from build123d import *

# Parameters (mm, degrees)
SKETCH_1_W          = 210
SKETCH_1_H          = 70
EXTRUDE_1_DEPTH     = 8
SKETCH_2_W          = 190
SKETCH_2_H          = 60
CUT_EXTRUDE_1_DEPTH = 10
SKETCH_3_R          = 1.5
CUT_EXTRUDE_2_DEPTH = 10
SKETCH_4_W          = 8
SKETCH_4_H          = 10
CUT_EXTRUDE_3_DEPTH = 5
FILLET_1_R          = 3


with BuildPart() as part:
    # 草图1 → 凸台-拉伸1 (new body)
    with BuildSketch(Plane.XY):
        with Locations((75, 11.5)):
            Rectangle(SKETCH_1_W, SKETCH_1_H)
    extrude(amount=EXTRUDE_1_DEPTH)

    # 草图2 → 切除-拉伸1 (cut)
    with BuildSketch(Plane.XY):
        with Locations((75, 11.5)):
            Rectangle(SKETCH_2_W, SKETCH_2_H)
    extrude(amount=CUT_EXTRUDE_1_DEPTH, mode=Mode.SUBTRACT)

    # 草图3 → 切除-拉伸2 (cut)
    with BuildSketch(Plane.XY):
        with Locations((-25, 36.5)):
            Circle(SKETCH_3_R)
        with Locations((175, 36.5)):
            Circle(SKETCH_3_R)
        with Locations((-25, -13.5)):
            Circle(SKETCH_3_R)
        with Locations((175, -13.5)):
            Circle(SKETCH_3_R)
    extrude(amount=CUT_EXTRUDE_2_DEPTH, mode=Mode.SUBTRACT)

    # 草图4 → 切除-拉伸3 (cut)
    with BuildSketch(Plane(origin=(0, 46.5, 0), x_dir=(1, 0, 0), z_dir=(0, 1, 0))):
        with Locations((75, -5)):
            Rectangle(SKETCH_4_W, SKETCH_4_H)
    extrude(amount=-CUT_EXTRUDE_3_DEPTH, mode=Mode.SUBTRACT)

    # 圆角1
    fillet_1_edges = [part.edges().sort_by_distance(p)[0] for p in [
        (-30, 46.5, 4),
        (180, 46.5, 4),
        (180, -23.5, 4),
        (-30, -23.5, 4),
    ]]
    fillet(fillet_1_edges, radius=FILLET_1_R)


solid = part.part
Verification items for the finished model (mm, model axes). A direction names the side the tool comes from. Coordinates: 2 decimals unless noted, no trailing zeros. Write each loop counter-clockwise with the first axis right and the second up, starting at its lowest first coordinate (ties: lowest second). Pieces come first, ordered by that corner, then holes. Notation, with made-up numbers: (-34.75, -22.75) -> (9.25, -22.75) arc R23 cw to (9.25, -9.75) -> close; hole circle Ø11 at (-23.5, 16). An arc over 180 degrees is marked (long way). One line per item, written item: value. Start each with the question number.
Q1. Mould release check, pull along X, two halves, no side actions. Record for faces 4 (the flat face through (79, 44, 4)), 5 (the flat face through (74, -23.5, 4)), 6 (the flat face through (-30, 11, 4)): pulls with the +X half, pulls with the -X half, needs draft (parallel to the pull), parting line crosses it, or undercut.
Q2. Cross-section at A-A on x = 14. Enter the section's corners in (y, z), and give its area (3 significant figures).
Q3. Cross-section at B-B on z = 5.5. Enter the section's corners in (x, y), and give its area (3 significant figures).
Q4. Access from +Z, -Z, +X, -X, +Y, -Y to the whole of each face (thin tool, end or side, straight path). Record for faces 1 (the flat face through (180, 11, 4)), 2 (the flat face through (74, -18.5, 4)), 3 (the flat face through (71, 44, 4)).
Q5. Thickness scan on L1, parallel to X at y = -13.5, z = 2.75; L2, parallel to Y at x = -25, z = 2.25; L3, parallel to X at y = 18, z = 4.25. Record the ranges inside material, lowest first. Write a range as from..to.
Q6. Go/stop test with flat-tipped pins: P1, Ø2.5, axis at x = -25, y = 36.5, coming from the -Z side; P2, Ø2.5, axis at y = 45, z = 5.5, coming from the -X side. Record where each tip stops, or that it passes through.
Q7. Cross-section at C-C on y = 15.5. Enter the section's corners in (x, z).
Checked values:
1. face 4: undercut
1. face 5: needs draft
1. face 6: pulls with the -X half
2. outline: (-23.5, 0) -> (-18.5, 0) -> (-18.5, 8) -> (-23.5, 8) -> close; (41.5, 0) -> (46.5, 0) -> (46.5, 8) -> (41.5, 8) -> close
2. area: 80.0 mm²
3. outline: (-30, -20.5) arc R3 ccw to (-27, -23.5) -> (177, -23.5) arc R3 ccw to (180, -20.5) -> (180, 43.5) arc R3 ccw to (177, 46.5) -> (79, 46.5) -> (79, 41.5) -> (170, 41.5) -> (170, -18.5) -> (-20, -18.5) -> (-20, 41.5) -> (71, 41.5) -> (71, 46.5) -> (-27, 46.5) arc R3 ccw to (-30, 43.5) -> close; hole circle Ø3 at (-25, -13.5); hole circle Ø3 at (-25, 36.5); hole circle Ø3 at (175, -13.5); hole circle Ø3 at (175, 36.5)
3. area: 3,220 mm²
4. face 1: +Z, -Z, +X, +Y, -Y
4. face 2: +Z, -Z
4. face 3: +Z, -Z, +Y
5. L1: x = -30..-26.5, -23.5..-20, 170..173.5, 176.5..180
5. L2: y = -23.5..-15, -12..35, 38..46.5
5. L3: x = -30..-20, 170..180
6. P1: passes through
6. P2: stops at x = -29.99
7. outline: (-30, 0) -> (-20, 0) -> (-20, 8) -> (-30, 8) -> close; (170, 0) -> (180, 0) -> (180, 8) -> (170, 8) -> close
